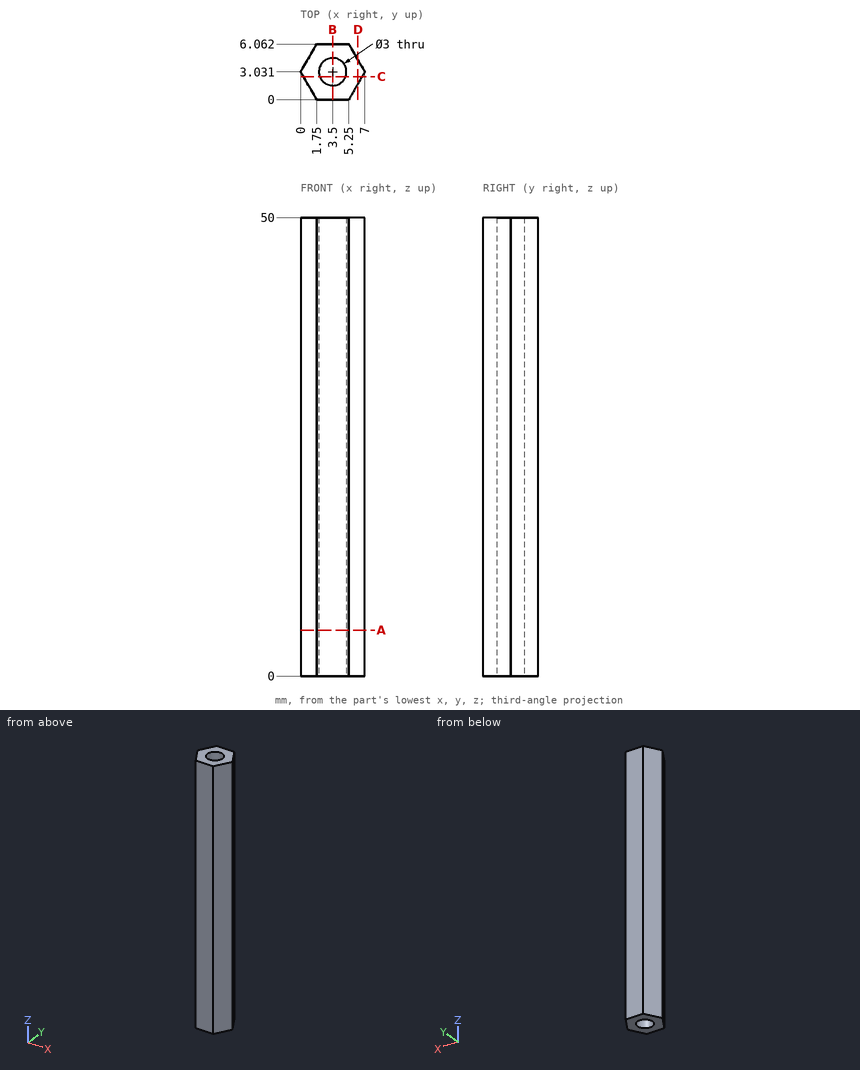
Could you check a few things on this drawing? It's one solid part, dimensions in mm from its lowest x, y, z. Coordinates: 2 decimals unless noted, no trailing zeros. Order: outer loops, then holes, each group sorted by start corner. A loop starts at its lowest first (then second) coordinate and runs counter-clockwise, first axis right, second up. Notation, with made-up numbers: (0.25, 4.25) - (30.25, 4.25) arc R24 ccw to (30.25, 26.25) - close; hole circle Ø5 at (-13.75, -29.5). An arc over 180 degrees is marked (long way). Answer as a JSON object with one key per item and string values. Group by question number.
Q1. Imagine slicing it at C-C (y = 2.5). Please give me the cut outline in (x, z).
Q2. Imagine slicing it at D-D (x = 6.25). Please give me the cut outline in (y, z), and give its area (3 significant figures).
Q3. I need wall thicknesses on line 1 (Y direction, x = 3.5, z = 35); line 2 (X direction, y = 4.25, z = 24) (1 decimal); line 3 (X direction, y = 2.5, z = 31.5). Which ranges of each line are inside material? Lowest first, please. Write a range as from..to.
Q4. Imagine slicing it at A-A (z = 5). Please give me the cut outline in (x, y).
Q5. Will these pins go through, and if not, where does the flat tip stop? P1, Ø1, axis at y = 4.5, z = 13, coming from the -X side; P2, Ø1, axis at y = 2, z = 21, coming from the -X side; P3, Ø3, axis at y = 5, z = 12, coming from the +X side; P4, Ø3.5, axis at x = 3.5, y = 3.03, coming from the -Z side.
Q6. Imagine slicing it at B-B (x = 3.5). Please give me the cut outline in (y, z), and give its area (3 significant figures).
Determined:
{
 "1": {"outline": "(0.31, 0) - (2.1, 0) - (2.1, 50) - (0.31, 50) - close; (4.9, 0) - (6.69, 0) - (6.69, 50) - (4.9, 50) - close"},
 "2": {"outline": "(1.73, 0) - (4.33, 0) - (4.33, 50) - (1.73, 50) - close", "area": "130 mm2"},
 "3": {"line 1": "y = 0..1.53, 4.53..6.06", "line 2": "x = 0.7..2.6, 4.4..6.3", "line 3": "x = 0.31..2.1, 4.9..6.69"},
 "4": {"outline": "(0, 3.03) - (1.75, 0) - (5.25, 0) - (7, 3.03) - (5.25, 6.06) - (1.75, 6.06) - close; hole circle Ø3 at (3.5, 3.03)"},
 "5": {"P1": "stops at x = 0.56", "P2": "stops at x = 0.31", "P3": "stops at x = 6.73", "P4": "stops at z = 0"},
 "6": {"outline": "(0, 0) - (1.53, 0) - (1.53, 50) - (0, 50) - close; (4.53, 0) - (6.06, 0) - (6.06, 50) - (4.53, 50) - close", "area": "153 mm2"}
}
